from build123d import *

# Parameters (mm, degrees)
SKETCH_1_W      = 13
SKETCH_1_H      = 11
SKETCH_1_R      = 2.5
SKETCH_1_W_2    = 6
SKETCH_1_H_2    = 7.5
EXTRUDE_1_DEPTH = 6
SKETCH_2_W      = 6
SKETCH_2_H      = 11
EXTRUDE_2_DEPTH = 5


with BuildPart() as part:
    # 草图1 → 凸台-拉伸1 (new body)
    with BuildSketch(Plane.XY):
        with Locations((5.75, 3.75)):
            Rectangle(SKETCH_1_W, SKETCH_1_H)
        with Locations((9, 3.75)):
            Circle(SKETCH_1_R, mode=Mode.SUBTRACT)
        with Locations((3, 3.75)):
            Rectangle(SKETCH_1_W_2, SKETCH_1_H_2, mode=Mode.SUBTRACT)
    extrude(amount=EXTRUDE_1_DEPTH)

    # 草图2 → 凸台-拉伸2 (add)
    with BuildSketch(Plane(origin=(12.25, 0, 0), x_dir=(0, 0, -1), z_dir=(1, 0, 0))):
        with Locations((-3, 3.75)):
            Rectangle(SKETCH_2_W, SKETCH_2_H)
    extrude(amount=EXTRUDE_2_DEPTH)


solid = part.part
Geometry check sheet. Reference: the model listing, model coordinates, mm. A direction names the side the tool comes from. Round coordinates to 2 decimals unless told otherwise and drop trailing zeros. Order: outer loops, then holes, each group sorted by start corner. A loop starts at its lowest first (then second) coordinate and runs counter-clockwise, first axis right, second up. Notation, with made-up numbers: (35.5, 38) - (89.5, 38) arc R9 ccw to (89.5, 49) - close; hole circle Ø9 at (-31, 68.25). An arc over 180 degrees is marked (long way). One line per question, with ' | ' between items. Start each with the question number.
(1) Sectioned sample at C-C on z = 1.45. Record the cut outline in (x, y).
(2) Release check for a two-part mould opening along Y. For faces 3 (the flat face through (0, 4, 3)), 4 (the flat face through (8, -1.75, 3)), 5 (the flat face through (17.25, 4, 3)), 6 (the flat face through (3, 7.5, 3)) record: released by +Y, released by -Y, zero draft, split by the parting line, or undercut.
(3) Sectioned sample at B-B on y = 3.75. Record the cut outline in (x, z).
(4) Depth check by flat-ended pin: pin 1 Ø3 at (x, y) = (9, 3.75) entering from -Z. Enter the tip coordinate at first touch or a pass-through.
(5) Thickness scan on L1, parallel to Y at x = 9, z = 2; L2, parallel to X at y = 2.5, z = 2.75; L3, parallel to Y at x = 4.5, z = 1.05. Record the ranges inside material, lowest first. Write a range as [from, to].
(6) Sectioned sample at D-D on y = 7. Record the cut outline in (x, z).
(7) Sectioned sample at A-A on x = 9. Record the cut outline in (y, z).
(8) Access from +Z, -Z, +X, -X, +Y, -Y to the whole of each face (thin tool, end or side, straight path). Record for faces 1 (the flat face through (3, 0, 3)), 2 (the flat face through (12, 4, 0)).
Conclusion:
1) outline: (-0.75, -1.75) - (17.25, -1.75) - (17.25, 9.25) - (-0.75, 9.25) - close; hole (0, 0) - (6, 0) - (6, 7.5) - (0, 7.5) - close; hole circle Ø5 at (9, 3.75)
2) face 3: undercut | face 4: released by -Y | face 5: zero draft | face 6: undercut
3) outline: (-0.75, 0) - (0, 0) - (0, 6) - (-0.75, 6) - close; (6, 0) - (6.5, 0) - (6.5, 6) - (6, 6) - close; (11.5, 0) - (17.25, 0) - (17.25, 6) - (11.5, 6) - close
4) pin 1: passes through
5) L1: y = [-1.75, 1.25], [6.25, 9.25] | L2: x = [-0.75, 0], [6, 6.83], [11.17, 17.25] | L3: y = [-1.75, 0], [7.5, 9.25]
6) outline: (-0.75, 0) - (0, 0) - (0, 6) - (-0.75, 6) - close; (6, 0) - (17.25, 0) - (17.25, 6) - (6, 6) - close
7) outline: (-1.75, 0) - (1.25, 0) - (1.25, 6) - (-1.75, 6) - close; (6.25, 0) - (9.25, 0) - (9.25, 6) - (6.25, 6) - close
8) face 1: +Z, -Z | face 2: -Z, +X, -X, +Y, -Y
